```python
from build123d import *

# Parameters (mm, degrees)
SKETCH1_R           = 1.65
BOSS_EXTRUDE1_DEPTH = 5.842
FILLET1_R           = 5
SKETCH2_R           = 1.5
CUT_EXTRUDE1_DEPTH  = 53.651011044


with BuildPart() as part:
    # Sketch1 → Boss-Extrude1 (new body)
    with BuildSketch(Plane.XY):
        with BuildLine():
            Line((-12.7, 0), (-12.7, 34.752122237))
            ThreePointArc((-12.7, 34.752122237), (0, -37), (12.7, 34.752122237))
            Line((12.7, 34.752122237), (12.7, 0))
            ThreePointArc((12.7, 0), (0, -12.7), (-12.7, 0))
        make_face()
        with Locations((22, 0)):
            Circle(SKETCH1_R, mode=Mode.SUBTRACT)
        with Locations((0, -22)):
            Circle(SKETCH1_R, mode=Mode.SUBTRACT)
        with Locations((-22, 0)):
            Circle(SKETCH1_R, mode=Mode.SUBTRACT)
    extrude(amount=BOSS_EXTRUDE1_DEPTH)

    # Fillet1
    fillet1_edges = [part.edges().sort_by_distance(p)[0] for p in [
        (12.7, 34.752122237, 2.921),
        (-12.7, 34.752122237, 2.921),
    ]]
    fillet(fillet1_edges, radius=FILLET1_R)

    # Sketch2 → Cut-Extrude1 (cut, through all)
    with BuildSketch(Plane.XY.offset(5.842)):
        with Locations((-15.556349186, -15.556349186)):
            Circle(SKETCH2_R)
        with Locations((-15.556349186, 15.556349186)):
            Circle(SKETCH2_R)
        with Locations((15.556349186, 15.556349186)):
            Circle(SKETCH2_R)
        with Locations((15.556349186, -15.556349186)):
            Circle(SKETCH2_R)
    extrude(amount=-CUT_EXTRUDE1_DEPTH, mode=Mode.SUBTRACT)


solid = part.part
```
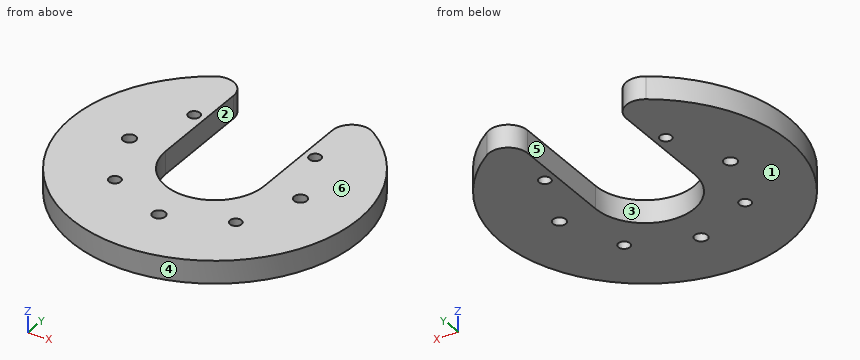
Work out the finished part from the listing and answer in its coordinate system (mm). Face numbers are marked on the shaded views. A direction names the side the tool comes from. Coordinates: 2 decimals unless noted, no trailing zeros. Order: outer loops, then holes, each group sorted by start corner. A loop starts at its lowest first (then second) coordinate and runs counter-clockwise, first axis right, second up. Notation, with made-up numbers: (-31.75, 63.5) - (-2.75, 63.5) arc R26 cw to (-2.75, 98.5) - close; hole circle Ø6 at (0.5, 84.5). An arc over 180 degrees is marked (long way). Answer as a JSON object with one key per item and string values.
1. Find section C-C on z = 4.75. Determine the outline of the cut face in (x, y).
Output values:
{"outline": "(-20.47, 30.82) arc R37 ccw (long way) to (20.47, 30.82) arc R5 ccw to (12.7, 26.66) - (12.7, 0) arc R12.7 cw to (-12.7, 0) - (-12.7, 26.66) arc R5 ccw to start; hole circle Ø3.3 at (-22, 0); hole circle Ø3 at (-15.56, -15.56); hole circle Ø3 at (-15.56, 15.56); hole circle Ø3.3 at (0, -22); hole circle Ø3 at (15.56, -15.56); hole circle Ø3 at (15.56, 15.56); hole circle Ø3.3 at (22, 0)"}
2. The mould has two halves that part along X. Classify the marked faces 1, 2, 3 and 4: +X half, -X half, draft (parallel to the pull), parting line (faces both ways), or undercut.
Output values:
{"face 1": "draft", "face 2": "undercut", "face 3": "undercut", "face 4": "parting line"}
3. Find section D-D on x = -19.5. Determine the outline of the cut face in (y, z).
Output values:
{"outline": "(-31.44, 0) - (31.32, 0) - (31.32, 5.84) - (-31.44, 5.84) - close"}
4. A tool of negligible diameter and unlimited length cuts with its end or side. For the marked faces 5 and 6, from which of +Z, -Z, +X, -X, +Y, -Y can it reach the whole face along a straight path? Write none if from no direction.
Output values:
{"face 5": "+Z, -Z, +Y", "face 6": "+Z, +X, -X, +Y, -Y"}
5. Each of these flat-tipped pins is pushed along its axis until it touches: P1, Ø3, axis at y = 11.5, z = 2.5, coming from the -X side; P2, Ø3, axis at y = 12.5, z = 2, coming from the +X side; P3, Ø1.8, axis at x = -15.56, y = -15.56, coming from the +Z side; P4, Ø1.5, axis at y = -1, z = 4, coming from the +X side. Where does it stop, or does it pass through?
Output values:
{"P1": "stops at x = -35.62", "P2": "stops at x = 35.33", "P3": "passes through", "P4": "stops at x = 37"}
6. Find section B-B on y = 12. Determine the outline of the cut face in (x, z).
Output values:
{"outline": "(-35, 0) - (-12.7, 0) - (-12.7, 5.84) - (-35, 5.84) - close; (12.7, 0) - (35, 0) - (35, 5.84) - (12.7, 5.84) - close"}
7. Consider line 1 (Y direction, x = 0, z = 3.6); line 2 (Y direction, x = 15, z = 1.2); line 3 (X direction, y = -15, z = 4.4). Determine where each line is inside the solid, lowest interval first.
Output values:
{"line 1": "y = -37 to -23.65, -20.35 to -12.7", "line 2": "y = -33.82 to -16.95, -14.16 to 14.16, 16.95 to 30.87", "line 3": "x = -33.82 to -16.95, -14.16 to 14.16, 16.95 to 33.82"}
8. Find section A-A on x = 0. Determine the outline of the cut face in (y, z), plus the area to 3 significant figures.
Output values:
{"outline": "(-37, 0) - (-23.65, 0) - (-23.65, 5.84) - (-37, 5.84) - close; (-20.35, 0) - (-12.7, 0) - (-12.7, 5.84) - (-20.35, 5.84) - close", "area": "123 mm²"}
